Part model, mm, in its own coordinate system. Round coordinates to 2 decimals unless told otherwise and drop trailing zeros. Order: outer loops, then holes, each group sorted by start corner. A loop starts at its lowest first (then second) coordinate and runs counter-clockwise, first axis right, second up. Notation, with made-up numbers: (57, 14) - (107, 14) arc R16 cw to (107, 44) - close; hole circle Ø7 at (-17, -7.75). An arc over 180 degrees is marked (long way). Answer as a JSON object with one key per item and string values.
```python
from build123d import *

# Parameters (mm, degrees)
AUFSATZ_LINEAR_AUSTRAGEN1_DEPTH = 0.25
AUFSATZ_LINEAR_AUSTRAGEN2_DEPTH = 0.5


with BuildPart() as part:
    # Skizze1 → Aufsatz-Linear austragen1 (new body, symmetric)
    with BuildSketch(Plane(origin=(0, 0, 0), x_dir=(1, 0, 0), z_dir=(0, 1, 0))):
        with BuildLine():
            Line((-36, 77.25), (-27, 77.25))
            ThreePointArc((-27, 77.25), (0, 73.25), (27, 77.25))
            Line((27, 77.25), (36, 77.25))
            Line((36, 77.25), (36, -59.75))
            ThreePointArc((36, -59.75), (32.045941546, -69.295941546), (22.5, -73.25))
            Line((22.5, -73.25), (-22.5, -73.25))
            ThreePointArc((-22.5, -73.25), (-32.045941546, -69.295941546), (-36, -59.75))
            Line((-36, -59.75), (-36, 77.25))
        make_face()
    extrude(amount=AUFSATZ_LINEAR_AUSTRAGEN1_DEPTH, both=True)

    # Skizze2 → Aufsatz-Linear austragen2 (add)
    with BuildSketch(Plane(origin=(0, 0.25, 0), x_dir=(1, 0, 0), z_dir=(0, 1, 0))):
        with BuildLine():
            Line((-35.998563753, -59.946917797), (-38, 77.25))
            Line((-38, 77.25), (-36, 77.25))
            Line((-36, 77.25), (-36, -59.75))
            ThreePointArc((-36, -59.75), (-35.999640933, -59.848461517), (-35.998563753, -59.946917797))
        make_face()
        with BuildLine():
            Line((36, 77.25), (36, -59.75))
            ThreePointArc((36, -59.75), (35.999640933, -59.848461517), (35.998563753, -59.946917797))
            Line((35.998563753, -59.946917797), (38, 77.25))
            Line((38, 77.25), (36, 77.25))
        make_face()
    extrude(amount=-AUFSATZ_LINEAR_AUSTRAGEN2_DEPTH)


solid = part.part
```
Item 1: Cut at A-A (y = 0.15). Write the cut outline in (x, z) (3 decimals).
Taken from the geometry:
{"outline": "(-38, -77.25) - (-27, -77.25) arc R93.125 cw to (27, -77.25) - (38, -77.25) - (35.999, 59.947) arc R13.5 ccw to (22.5, 73.25) - (-22.5, 73.25) arc R13.5 ccw to (-35.999, 59.947) - close"}
Item 2: Cut at C-C (x = 15). Write the cut outline in (y, z).
Taken from the geometry:
{"outline": "(-0.25, -74.47) - (0.25, -74.47) - (0.25, 73.25) - (-0.25, 73.25) - close"}
Item 3: Probe L1, parallel to Z at x = 1, y = 0.1; L2, parallel to Z at x = 23, y = 0.1; L3, parallel to X at y = -0.2, z = 5. List the from-to ranges inside material, lowest first. Write a range as from..to.
Taken from the geometry:
{"L1": "-73.26..73.25", "L2": "-76.13..73.24", "L3": "-36.8..36.8"}
Item 4: Cut at B-B (z = -14). Write the cut outline in (x, y).
Taken from the geometry:
{"outline": "(-37.08, -0.25) - (37.08, -0.25) - (37.08, 0.25) - (-37.08, 0.25) - close"}
